Check sheet for the drawn part. Datum: minimum x, y, z corner. Units: mm. A direction names the side the tool comes from. Give positions to 0.01 mm unless a question says otherwise; leave off trailing zeros. Write each loop counter-clockwise with the first axis right and the second up, starting at its lowest first coordinate (ties: lowest second). Pieces come first, ordered by that corner, then holes. Notation, with made-up numbers: (-19.75, 68) - (21.25, 68) arc R25 cw to (21.25, 85) - close; hole circle Ø11 at (74.25, -18). An arc over 180 degrees is marked (long way). One line per question, with ' | ' between items. Start each with the question number.
Q1. Release check for a two-part mould opening along Z. For the marked faces 3, 4, 5 and 6 record: +Z half, -Z half, draft (parallel to the pull), parting line (faces both ways), or undercut.
Q2. Section check C-C on z = 5. Record the boundary of the cut face in (x, y), and give its area (3 significant figures).
Q3. Thickness scan on L1, parallel to Z at x = 28, y = 0.9; L2, parallel to X at y = 1, z = 8.5; L3, parallel to Z at x = 2.75, y = 0.85. Record the ranges inside material, lowest first. Write a range as [from, to].
Q4. Set-up check for the marked faces 1 and 2: record each of +Z, -Z, +X, -X, +Y, -Y from which the full face is reachable in a straight line by a thin tool's end or side.
Q5. Gauge pin test, flat ends, axial feed: P1, Ø1, axis at x = 27, y = 1.5, coming from the -Z side; P2, Ø1, axis at y = 1.5, z = 10.5, coming from the -X side. Record the tip position at first contact, or that the pin passes through.
Q6. Section check B-B on y = 0.9. Record the boundary of the cut face in (x, z).
Q7. Section check A-A on z = 11.95. Record the boundary of the cut face in (x, y), and give its area (3 significant figures).
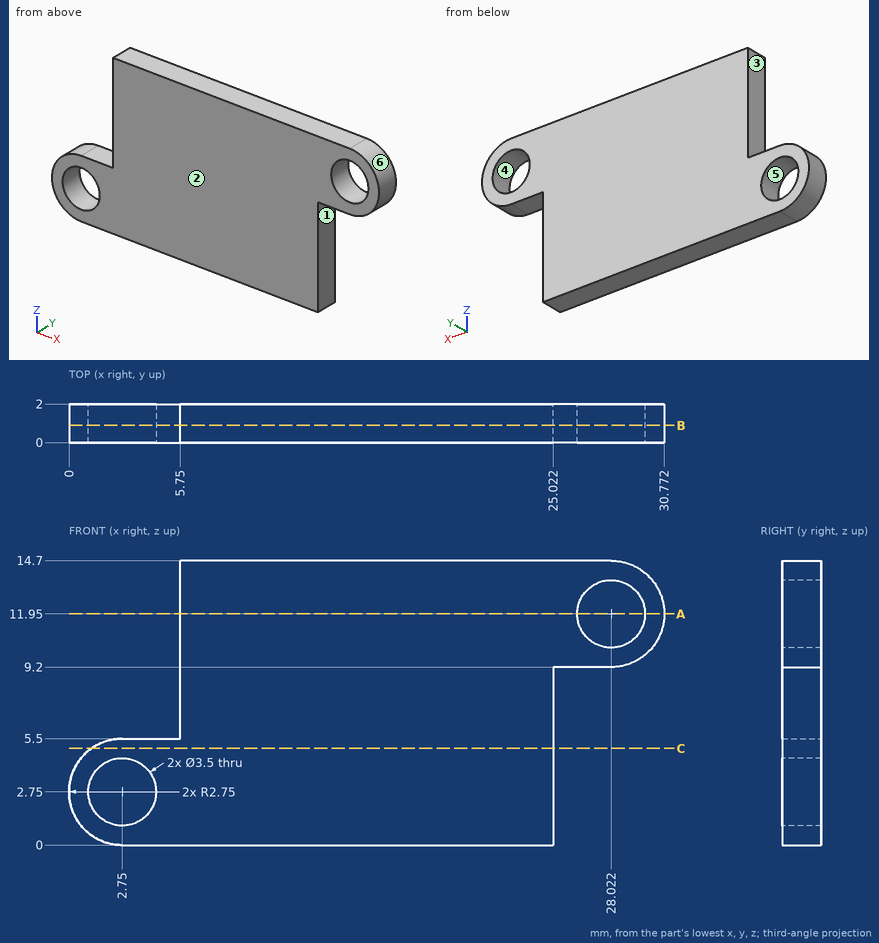
Working result:
1) face 3: draft | face 4: undercut | face 5: undercut | face 6: parting line
2) outline: (1.17, 0) - (25.02, 0) - (25.02, 2) - (1.17, 2) - close | area: 47.7 mm2
3) L1: z = [9.2, 10.2], [13.7, 14.7] | L2: x = [5.75, 25.02] | L3: z = [0, 1], [4.5, 5.5]
4) face 1: -Z, +X, +Y, -Y | face 2: +Z, -Z, +X, -X, -Y
5) P1: stops at z = 9.2 | P2: stops at x = 5.75
6) outline: (2.75, 0) - (25.02, 0) - (25.02, 9.2) - (28.02, 9.2) arc R2.75 ccw to (28.02, 14.7) - (5.75, 14.7) - (5.75, 5.5) - (2.75, 5.5) arc R2.75 ccw to start; hole circle Ø3.5 at (2.75, 2.75); hole circle Ø3.5 at (28.02, 11.95)
7) outline: (5.75, 0) - (26.27, 0) - (26.27, 2) - (5.75, 2) - close; (29.77, 0) - (30.77, 0) - (30.77, 2) - (29.77, 2) - close | area: 43.0 mm2
